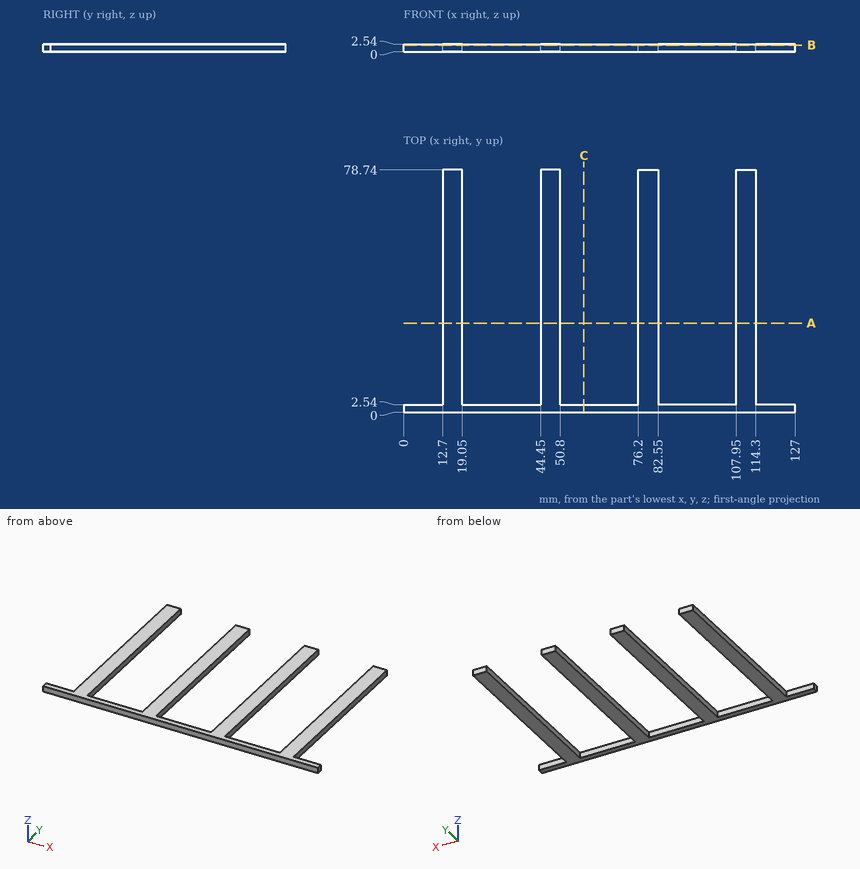
Print and shaded views of the part. All mm, measured from the part's lowest x, y and z. Coordinates: 2 decimals unless noted, no trailing zeros. Write each loop counter-clockwise with the first axis right and the second up, starting at its lowest first coordinate (ties: lowest second). Pieces come first, ordered by that corner, then holes. Notation, with made-up numbers: (28.5, 48) - (55.5, 48) arc R28 ccw to (55.5, 67) - close; hole circle Ø9 at (-9, -0.75). An arc over 180 degrees is marked (long way). One line per question, with ' | ' between items. Start each with the question number.
Q1. Drill centre lines: line 1 (X direction, y = 65.5, z = 1); line 2 (Y direction, x = 51, z = 1.2). Where is each one in solid material? Low to high. Write a range as [from, to].
Q2. Cut at B-B, the plane z = 2.15. List the corners of the cut face in (x, y), then the cut area to 3 significant figures.
Q3. Cut at A-A, the plane y = 29. List the corners of the cut face in (x, z), then the cut area to 3 significant figures.
Q4. Cut at C-C, the plane x = 58.5. List the corners of the cut face in (y, z).
Q5. Pin check, flat tips, straight feed: pin 1 (1.3 mm diameter, centred on x = 121, z = 1.5, fed in from +Y); pin 2 (1 mm diameter, centred on y = 16.5, z = 2, fed in from -X); pin 3 (8 mm diameter, centred on x = 85, y = 20, fed in from -Z); pin 4 (1.3 mm diameter, centred on y = 30.5, z = 1, fed in from +X). Stop position of each tip, or through.
Answer below:
1) line 1: [12.7, 19.05], [44.45, 50.8], [76.2, 82.55], [107.95, 114.3] | line 2: [0, 2.54]
2) outline: (0, 0) - (127, 0) - (127, 2.54) - (114.3, 2.54) - (114.3, 78.74) - (107.95, 78.74) - (107.95, 2.54) - (82.55, 2.54) - (82.55, 78.74) - (76.2, 78.74) - (76.2, 2.54) - (50.8, 2.54) - (50.8, 78.74) - (44.45, 78.74) - (44.45, 2.54) - (19.05, 2.54) - (19.05, 78.74) - (12.7, 78.74) - (12.7, 2.54) - (0, 2.54) - close | area: 2,260 mm^2
3) outline: (12.7, 0) - (19.05, 0) - (19.05, 2.54) - (12.7, 2.54) - close; (44.45, 0) - (50.8, 0) - (50.8, 2.54) - (44.45, 2.54) - close; (76.2, 0) - (82.55, 0) - (82.55, 2.54) - (76.2, 2.54) - close; (107.95, 0) - (114.3, 0) - (114.3, 2.54) - (107.95, 2.54) - close | area: 64.5 mm^2
4) outline: (0, 0) - (2.54, 0) - (2.54, 2.54) - (0, 2.54) - close
5) pin 1: y = 2.54 | pin 2: x = 12.7 | pin 3: z = 0 | pin 4: x = 114.3
